Source: CAD feature listing. Evaluate the final solid. Frame: model axes, mm. Give positions to 0.01 mm unless a question says otherwise; leave off trailing zeros. Write each loop counter-clockwise with the first axis right and the second up, starting at its lowest first coordinate (ties: lowest second). Pieces come first, ordered by that corner, then holes.
```python
from build123d import *

# Parameters (mm, degrees)
F1_DEPTH = 0.8
F2_R     = 3


with BuildPart() as f1:
    # F0 (on Top) → F1 (new body)
    with BuildSketch(Plane.XY):
        with BuildLine():
            Line((-40, 825), (-95, 825))
            ThreePointArc((-95, 825), (-98.535534, 823.535534), (-100, 820))
            Line((-100, 820), (-100, 801.5))
            Line((-100, 801.5), (-70, 801.5))
            ThreePointArc((-70, 801.5), (-68.93934, 801.06066), (-68.5, 800))
            ThreePointArc((-68.5, 800), (-68.93934, 798.93934), (-70, 798.5))
            Line((-70, 798.5), (-100, 798.5))
            Line((-100, 798.5), (-100, 771.5))
            Line((-100, 771.5), (-70, 771.5))
            ThreePointArc((-70, 771.5), (-68.93934, 771.06066), (-68.5, 770))
            ThreePointArc((-68.5, 770), (-68.93934, 768.93934), (-70, 768.5))
            Line((-70, 768.5), (-100, 768.5))
            Line((-100, 768.5), (-100, 351.5))
            Line((-100, 351.5), (-70, 351.5))
            ThreePointArc((-70, 351.5), (-68.93934, 351.06066), (-68.5, 350))
            ThreePointArc((-68.5, 350), (-68.93934, 348.93934), (-70, 348.5))
            Line((-70, 348.5), (-100, 348.5))
            Line((-100, 348.5), (-100, 321.5))
            Line((-100, 321.5), (-70, 321.5))
            ThreePointArc((-70, 321.5), (-68.93934, 321.06066), (-68.5, 320))
            ThreePointArc((-68.5, 320), (-68.93934, 318.93934), (-70, 318.5))
            Line((-70, 318.5), (-100, 318.5))
            Line((-100, 318.5), (-100, 31.5))
            Line((-100, 31.5), (-70, 31.5))
            ThreePointArc((-70, 31.5), (-68.93934, 31.06066), (-68.5, 30))
            ThreePointArc((-68.5, 30), (-68.93934, 28.93934), (-70, 28.5))
            Line((-70, 28.5), (-100, 28.5))
            Line((-100, 28.5), (-100, 1.5))
            Line((-100, 1.5), (-70, 1.5))
            ThreePointArc((-70, 1.5), (-68.93934, 1.06066), (-68.5, 0))
            ThreePointArc((-68.5, 0), (-68.93934, -1.06066), (-70, -1.5))
            Line((-70, -1.5), (-100, -1.5))
            Line((-100, -1.5), (-100, -20))
            ThreePointArc((-100, -20), (-98.535534, -23.535534), (-95, -25))
            Line((-95, -25), (-40, -25))
            ThreePointArc((-40, -25), (-11.715729, -13.284271), (0, 15))
            Line((0, 15), (0, 785))
            ThreePointArc((0, 785), (-11.715729, 813.284271), (-40, 825))
        make_face()
    extrude(amount=F1_DEPTH)

    # F2
    f2_edges = [f1.edges().sort_by_distance(p)[0] for p in [
        (-100, 801.5, 0.4),
        (-100, 798.5, 0.4),
        (-100, 771.5, 0.4),
        (-100, 768.5, 0.4),
        (-100, 351.5, 0.4),
        (-100, 348.5, 0.4),
        (-100, 321.5, 0.4),
        (-100, 318.5, 0.4),
        (-100, 31.5, 0.4),
        (-100, 28.5, 0.4),
        (-100, 1.5, 0.4),
        (-100, -1.5, 0.4),
    ]]
    fillet(f2_edges, radius=F2_R)


solid = f1.part
```
1. Line query: L1, parallel to X at y = 770.5, z = 0.3; L2, parallel to Y at x = -18, z = 0.15; L3, parallel to Y at x = -26, z = 0.1. Output: solid intervals per line, ascending.
2. Cut plane A-A, the plane x = -87. Return the cut outline in (y, z).
3. Cut plane B-B, the plane x = -8.5. Return the cut outline in (y, z), then the cut area to 3 significant figures.
Response values:
1. L1: x = -68.59 to 0
1. L2: y = -18.41 to 818.41
1. L3: y = -22.47 to 822.47
2. outline: (-25, 0) - (-1.5, 0) - (-1.5, 0.8) - (-25, 0.8) - close; (1.5, 0) - (28.5, 0) - (28.5, 0.8) - (1.5, 0.8) - close; (31.5, 0) - (318.5, 0) - (318.5, 0.8) - (31.5, 0.8) - close; (321.5, 0) - (348.5, 0) - (348.5, 0.8) - (321.5, 0.8) - close; (351.5, 0) - (768.5, 0) - (768.5, 0.8) - (351.5, 0.8) - close; (771.5, 0) - (798.5, 0) - (798.5, 0.8) - (771.5, 0.8) - close; (801.5, 0) - (825, 0) - (825, 0.8) - (801.5, 0.8) - close
3. outline: (-9.65, 0) - (809.65, 0) - (809.65, 0.8) - (-9.65, 0.8) - close
3. area: 655 mm2
